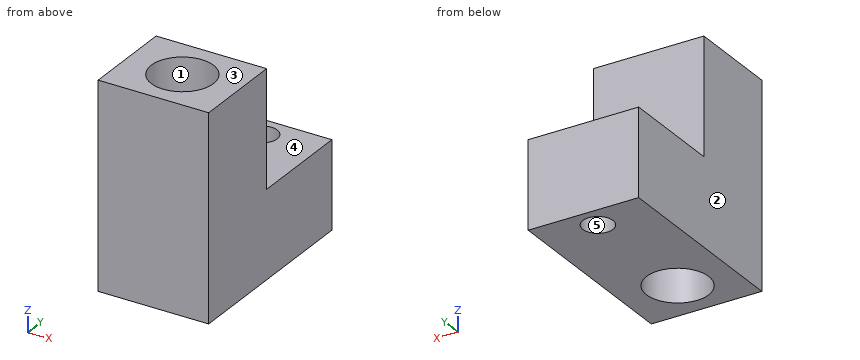
```python
from build123d import *

# Parameters (mm, degrees)
BOSS_EXTRUDE1_DEPTH          = 12.065
TAP_DRILL_FOR_M8X1_25_TAP1_D = 6.8
SKETCH6_R                    = 1.651
CUT_EXTRUDE2_DEPTH           = 34.251209752


with BuildPart() as part:
    # Sketch1 → Boss-Extrude1 (new body)
    with BuildSketch(Plane(origin=(0, 0, 0), x_dir=(0, 0, -1), z_dir=(1, 0, 0))):
        Polygon((0, 0), (0, 10.16), (12.7, 10.16), (12.7, 21.59), (22.225, 21.59), (22.225, 0), align=None)
    extrude(amount=-BOSS_EXTRUDE1_DEPTH)

    # Tap Drill for M8x1.25 Tap1 (through all)
    with Locations(Plane(origin=(-0.703177612, 1.547352974, -22.225), x_dir=(1, 0, 0), z_dir=(0, 0, -1))):
        with Locations((-5.329322388, -3.532647026)):
            Hole(TAP_DRILL_FOR_M8X1_25_TAP1_D / 2)

    # Sketch6 → Cut-Extrude2 (cut, through all)
    with BuildSketch(Plane(origin=(0, 0, -22.225), x_dir=(-1, 0, 0), z_dir=(0, 0, -1))):
        with Locations(Location((6.0325, 19.05, 0), (0, 0, 90))):
            Circle(SKETCH6_R)
    extrude(amount=-CUT_EXTRUDE2_DEPTH, mode=Mode.SUBTRACT)


solid = part.part
```
Could you check a few things on this model? Use its own coordinates, in mm. Face numbers are marked on the shaded views. A direction names the side the tool comes from. Give positions to 0.01 mm unless a question says otherwise; leave off trailing zeros. Order: outer loops, then holes, each group sorted by start corner. A loop starts at its lowest first (then second) coordinate and runs counter-clockwise, first axis right, second up.
Q1. I'm going to push a flat-ended pin straight in: P1, Ø1, axis at x = -8.5, y = 13.5, coming from the +Z side. Where does the tip first touch, or does it pass through?
Q2. We'd pull the mould along X, two halves only. Please class the marked faces 1, 2 and 3: +X half, -X half, draft (parallel to the pull), parting line (faces both ways), or undercut.
Q3. If I drill on line 1 along X through (y, z) = (19.05, -16) (1 decimal); line 2 along Y through (x, z) = (-6.25, -19); line 3 along Y through (x, z) = (-6.25, -4.5), over which ranges is the centre line in solid material (lowest first)?
Q4. Suppose I cut it at D-D, the plane x = -5.25. Write out the boundary of the cut face in (y, z) (3 decimals).
Q5. For the marked faces 4 and 5, which set-ups out of +Z, -Z, +X, -X, +Y, -Y let a thin tool reach every point of the face, with its end or its side?
Q6. Suppose I cut it at A-A, the plane y = 19.05. Write out the boundary of the cut face in (x, z) (1 decimal).
Q7. Suppose I cut it at C-C, the plane y = 5.08. Write out the boundary of the cut face in (x, z) (1 decimal).
Q8. Suppose I cut it at B-B, the plane z = -3. Write out the boundary of the cut face in (x, y) (1 decimal).
Solution:
1. P1: stops at z = -12.7
2. face 1: undercut
2. face 2: -X half
2. face 3: draft
3. line 1: x = -12.1 to -7.7, -4.4 to 0
3. line 2: y = 0 to 1.69, 8.47 to 17.41, 20.69 to 21.59
3. line 3: y = 0 to 1.69, 8.47 to 10.16
4. outline: (0, -22.225) - (1.771, -22.225) - (1.771, 0) - (0, 0) - close; (8.389, -22.225) - (17.596, -22.225) - (17.596, -12.7) - (10.16, -12.7) - (10.16, 0) - (8.389, 0) - close; (20.504, -22.225) - (21.59, -22.225) - (21.59, -12.7) - (20.504, -12.7) - close
5. face 4: +Z, +X, -X, +Y
5. face 5: +Z, -Z
6. outline: (-12.1, -22.2) - (-7.7, -22.2) - (-7.7, -12.7) - (-12.1, -12.7) - close; (-4.4, -22.2) - (0, -22.2) - (0, -12.7) - (-4.4, -12.7) - close
7. outline: (-12.1, -22.2) - (-9.4, -22.2) - (-9.4, 0) - (-12.1, 0) - close; (-2.6, -22.2) - (0, -22.2) - (0, 0) - (-2.6, 0) - close
8. outline: (-12.1, 0) - (0, 0) - (0, 10.2) - (-12.1, 10.2) - close; hole circle Ø6.8 at (-6, 5.1)
